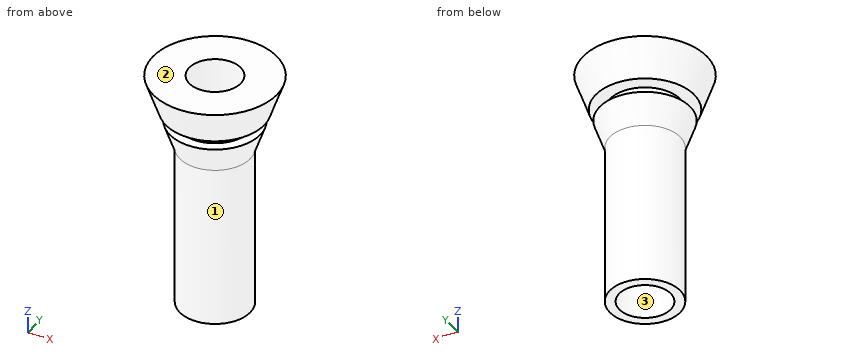
```python
from build123d import *

# Parameters (mm, degrees)
CYLINDER043_R     = 2.7
CYLINDER043_DEPTH = 25
CYLINDER042_R     = 3.7
CYLINDER042_DEPTH = 25
CYLINDER040_R     = 3.7
CYLINDER040_DEPTH = 1.2
CYLINDER041_R     = 6
CYLINDER041_DEPTH = 1.2


with BuildPart() as cylinder041:
    # Cylinder043 → Cylinder043 (new body)
    with BuildSketch(Plane.XY.offset(-38)):
        Circle(CYLINDER043_R)
    extrude(amount=CYLINDER043_DEPTH)


with BuildPart() as cylinder040:
    # Cylinder042 → Cylinder042 (new body)
    with BuildSketch(Plane.XY.offset(-38)):
        Circle(CYLINDER042_R)
    extrude(amount=CYLINDER042_DEPTH)


with BuildPart() as cylinder038:
    # Cylinder040 → Cylinder040 (new body)
    with BuildSketch(Plane.XY.offset(-18)):
        Circle(CYLINDER040_R)
    extrude(amount=CYLINDER040_DEPTH)


with BuildPart() as cut013005:
    # Cylinder041 → Cylinder041 (new body)
    with BuildSketch(Plane.XY.offset(-18)):
        Circle(CYLINDER041_R)
    extrude(amount=CYLINDER041_DEPTH)

    # Cut013005: cut Cylinder038
    add(cylinder038.part, mode=Mode.SUBTRACT)


with BuildPart() as connector_boot:
    # Cone004 → Cone004 (revolve)
    with BuildSketch(Plane(origin=(0, 0, -21), x_dir=(1, 0, 0), z_dir=(0, -1, 0))):
        Polygon((0, 0), (3.7, 0), (6.5, 8), (0, 8), align=None)
    revolve(axis=Axis((0, 0, -21), (0, 0, 1)))

    # Cut013006: cut Cut013005
    add(cut013005.part, mode=Mode.SUBTRACT)

    # Fusion017: union Cylinder040
    add(cylinder040.part)

    # Cut013007: cut Cylinder041
    add(cylinder041.part, mode=Mode.SUBTRACT)


with BuildPart() as connector_boot_1:
    # Cut013007 placement: moved
    add(connector_boot.part.moved(Location((0, 0, -15))))


solid = connector_boot_1.part
```
Input: part model. Units: mm. Frame: model coordinates. Face numbers are marked on the shaded views. Give positions to 0.01 mm unless a question says otherwise; leave off trailing zeros. Loops run counter-clockwise (first coordinate to the right, second up) from the corner with the lowest first, then second, coordinate; pieces in that order, holes last. Notation, with made-up numbers: M 57.25,53.5 L 88.25,53.5 A34 ccw 88.25,92.5 Z; hole C 55,47 d8. An arc over 180 degrees is marked long. Answer as CSV lines item,"result". Start each with the question number.
1. Section D-D on z = -34.5. Return loops of the section in (x, y) (3 decimals), plus the area to 3 significant figures.
2. Section C-C on z = -50.75. Return loops of the section in (x, y), plus the area to 3 significant figures.
3. Line query: L1, parallel to Y at x = 0, z = -40; L2, parallel to X at y = -0.5, z = -30; L3, parallel to Z at x = -1, y = -4.75. Output: solid intervals per line, ascending.
4. Pull-direction query (X, two-part tool) for the marked faces 1, 2 and 3; classes: released by +X, released by -X, zero draft, split by the parting line, or undercut.
5. Section A-A on x = 0. Return loops of the section in (y, z).
6. Pin query (flat end, axial travel): P1, Ø4, axis at x = -3, z = -35.5, coming from the +Y side; P2, Ø5, axis at x = -0.5, y = -0.5, coming from the +Z side; P3, Ø6, axis at y = 2.5, z = -50, coming from the +X side; P4, Ø4, axis at y = -3, z = -35, coming from the +X side. Return the tip coordinate at first contact, or that it passes through.
Computed values:
1,outline,"C 0,0 d8.45; hole C 0,0 d5.4"
1,area,"33.2 mm²"
2,outline,"C 0,0 d7.4; hole C 0,0 d5.4"
2,area,"20.1 mm²"
3,L1,"y = -3.7 to -2.7, 2.7 to 3.7"
3,L2,"x = -5.78 to -2.65, 2.65 to 5.78"
3,L3,"z = -31.8 to -28"
4,face 1,"split by the parting line"
4,face 2,"zero draft"
4,face 3,"undercut"
5,outline,"M -6.5,-28 L -5.17,-31.8 L -3.7,-31.8 L -3.7,-33 L -4.75,-33 L -3.7,-36 L -3.7,-53 L -2.7,-53 L -2.7,-28 Z; M 2.7,-53 L 3.7,-53 L 3.7,-36 L 4.75,-33 L 3.7,-33 L 3.7,-31.8 L 5.17,-31.8 L 6.5,-28 L 2.7,-28 Z"
6,P1,"stops at y = 4.07"
6,P2,"stops at z = -28"
6,P3,"stops at x = 3.7"
6,P4,"stops at x = 4.26"
